Design review of the part shown in the three views and the two pictorial views. Dimensions are in mm from the part's minimum x, y and z. A direction names the side the tool comes from. Round coordinates to 2 decimals unless told otherwise and drop trailing zeros. Loops run counter-clockwise (first coordinate to the right, second up) from the corner with the lowest first, then second, coordinate; pieces in that order, holes last.
1) Insertion check: pin 1 (2.5 mm diameter, centred on y = 37.5, z = 37.5, fed in from -X); pin 2 (8 mm diameter, centred on x = 59, y = 30, fed in from -Z); pin 3 (2.5 mm diameter, centred on y = 36.65, z = 36.65, fed in from -X); pin 4 (6 mm diameter, centred on y = 13, z = 29.5, fed in from -X). Each pin has a flat end and moves straight along its axis. Give the tip position at first contact, or say it passes through.
2) Take a section at A-A (z = 36.65). State the section outline as (x, y) points.
3) Take a section at D-D (y = 30.5). State the section outline as (x, z) points.
4) Tool access review of the marked faces 1 and 2: name each direction out of +Z, -Z, +X, -X, +Y, -Y from which nothing blocks a thin tool from reaching the whole face with its end or side.
5) Take a section at B-B (y = 22). State the section outline as (x, z) points.
6) Take a section at C-C (x = 15.5). State the section outline as (y, z) points, then the cut area to 3 significant figures.
7) Wall thickness on L1, parallel to Z at x = 29.3, y = 36.65; L2, parallel to Z at x = 27, y = 5: over which ranges is each line inside the solid? List them lowest first.
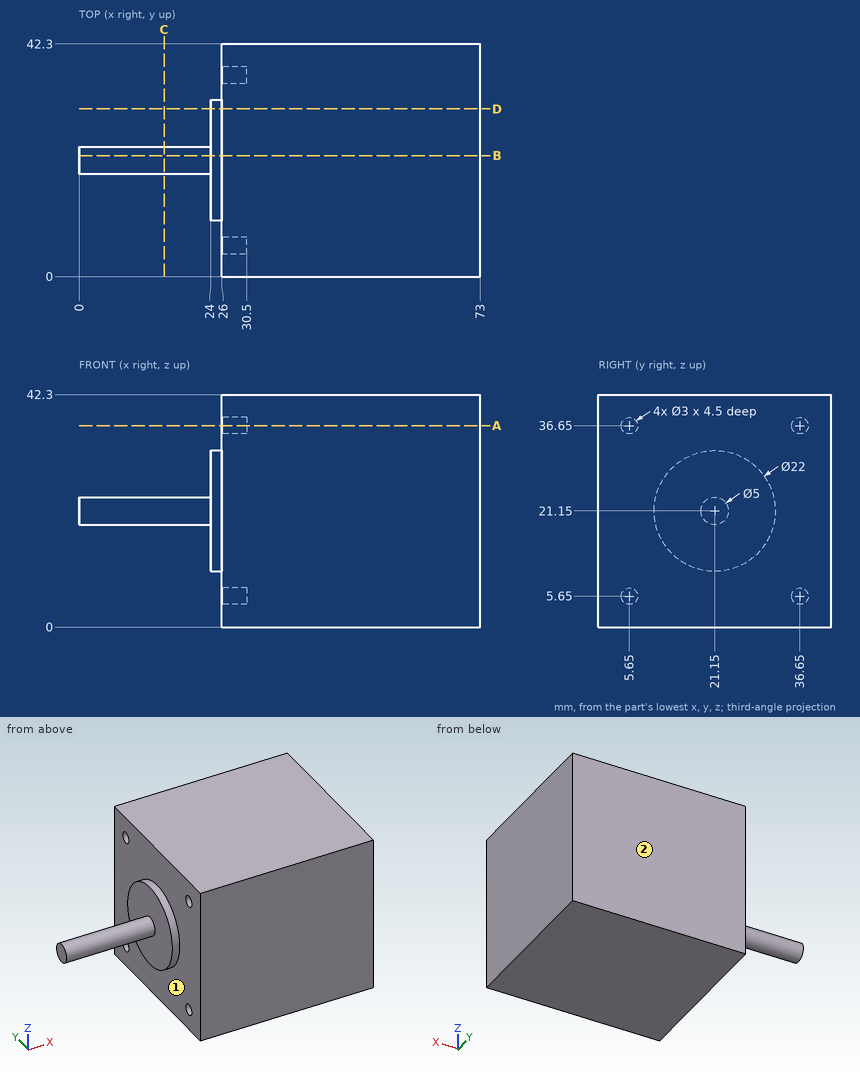
Response:
1. pin 1: stops at x = 26
1. pin 2: stops at z = 0
1. pin 3: stops at x = 30.5
1. pin 4: stops at x = 24
2. outline: (26, 0) - (73, 0) - (73, 42.3) - (26, 42.3) - (26, 38.15) - (30.5, 38.15) - (30.5, 35.15) - (26, 35.15) - (26, 7.15) - (30.5, 7.15) - (30.5, 4.15) - (26, 4.15) - close
3. outline: (24, 15.36) - (26, 15.36) - (26, 0) - (73, 0) - (73, 42.3) - (26, 42.3) - (26, 26.94) - (24, 26.94) - close
4. face 1: -X
4. face 2: +Z, -Z, +X, -X, +Y
5. outline: (0, 18.8) - (24, 18.8) - (24, 10.18) - (26, 10.18) - (26, 0) - (73, 0) - (73, 42.3) - (26, 42.3) - (26, 32.12) - (24, 32.12) - (24, 23.5) - (0, 23.5) - close
6. outline: circle Ø5 at (21.15, 21.15)
6. area: 19.6 mm2
7. L1: z = 0 to 4.15, 7.15 to 35.15, 38.15 to 42.3
7. L2: z = 0 to 4.3, 7 to 35.3, 38 to 42.3
